from build123d import *

# Parameters (mm, degrees)
SHAPE_DEPTH         = 10.75
CUT_EXTRUDE1_DEPTH  = 6.75
CUT_EXTRUDE2_REACH  = 6
FILLET1_R           = 0.2
SKETCH4_R           = 1
BOSS_EXTRUDE2_DEPTH = 6.1
FILLET2_R           = 1
SKETCH5_W           = 0.2
SKETCH5_H           = 2
SKETCH5_W_2         = 2
SKETCH5_H_2         = 0.2
CUT_EXTRUDE3_DEPTH  = 6.75
CUT_EXTRUDE4_DEPTH  = 2.4
CUT_EXTRUDE5_DEPTH  = 1
SKETCH7_R           = 1.225
SKETCH7_R_2         = 0.625
BOSS_EXTRUDE3_DEPTH = 4
SKETCH9_W           = 1.225
SKETCH9_H           = 2.45
CUT_EXTRUDE6_DEPTH  = 2.3


with BuildPart() as part:
    # Sketch1 → Shape (new body)
    with BuildSketch(Plane(origin=(0, 0, 0), x_dir=(1, 0, 0), z_dir=(0, 1, 0))):
        Polygon((5.075, -1.6), (5.075, 1.6), (4.075, 2.6), (-5.075, 2.6), (-5.075, -2.6), (4.075, -2.6), align=None)
    extrude(amount=SHAPE_DEPTH)

    # Sketch2 → Cut-Extrude1 (cut)
    with BuildSketch(Plane(origin=(0, 10.75, 0), x_dir=(1, 0, 0), z_dir=(0, 1, 0))):
        Polygon((3.826471863, -2), (4.475, -1.351471863), (4.475, 1.351471863), (3.826471863, 2), (-4.475, 2), (-4.475, -2), align=None)
    extrude(amount=-CUT_EXTRUDE1_DEPTH, mode=Mode.SUBTRACT)

    # Sketch3 → Cut-Extrude2 (cut, up to next)
    with BuildSketch(Plane(origin=(0, 4, 0), x_dir=(1, 0, 0), z_dir=(0, 1, 0)), mode=Mode.PRIVATE) as cut_extrude2_sk1:
        with BuildLine():
            Line((-1.675378875, -1.6), (1.675378875, -1.6))
            ThreePointArc((1.675378875, -1.6), (0.7, 0), (1.675378875, 1.6))
            Line((1.675378875, 1.6), (-1.675378875, 1.6))
            ThreePointArc((-1.675378875, 1.6), (-0.963068312, 0.936931688), (-0.7, 0))
            ThreePointArc((-0.7, 0), (-0.963068312, -0.936931688), (-1.675378875, -1.6))
        make_face()
    cut_extrude2_tool1 = extrude(cut_extrude2_sk1.sketch, amount=-CUT_EXTRUDE2_REACH, mode=Mode.PRIVATE) & part.part
    add(cut_extrude2_tool1.solids().sort_by_distance((0, 4, 0))[0], mode=Mode.SUBTRACT)

    # Fillet1
    fillet1_edges = [part.edges().sort_by_distance(p)[0] for p in [
        (1.675378875, 2, 1.6),
        (-1.675378875, 2, 1.6),
        (-1.675378875, 2, -1.6),
        (1.675378875, 2, -1.6),
    ]]
    fillet(fillet1_edges, radius=FILLET1_R)

    # Sketch4 → Boss-Extrude2 (add)
    with BuildSketch(Plane(origin=(0, 4, 0), x_dir=(1, 0, 0), z_dir=(0, 1, 0))):
        with Locations((-2.5, 0)):
            Circle(SKETCH4_R)
        with Locations((2.5, 0)):
            Circle(SKETCH4_R)
    extrude(amount=BOSS_EXTRUDE2_DEPTH)

    # Fillet2
    fillet2_edges = [part.edges().sort_by_distance(p)[0] for p in [
        (-3.5, 10.1, 0),
        (1.5, 10.1, 0),
    ]]
    fillet(fillet2_edges, radius=FILLET2_R)

    # Sketch5 → Cut-Extrude3 (cut)
    with BuildSketch(Plane(origin=(0, 10.75, 0), x_dir=(1, 0, 0), z_dir=(0, 1, 0))):
        with Locations((-2.5, 0)):
            Rectangle(SKETCH5_W, SKETCH5_H)
        with Locations((-2.5, 0)):
            Rectangle(SKETCH5_W_2, SKETCH5_H_2)
        with Locations((2.5, 0)):
            Rectangle(SKETCH5_W_2, SKETCH5_H_2)
        with Locations((2.5, 0)):
            Rectangle(SKETCH5_W, SKETCH5_H)
    extrude(amount=-CUT_EXTRUDE3_DEPTH, mode=Mode.SUBTRACT)

    # Sketch6 → Cut-Extrude4 (cut)
    with BuildSketch(Plane(origin=(0, 0.5, 0), x_dir=(-1, 0, 0), z_dir=(0, -1, 0))):
        Polygon((-5.075, -1.6), (-4.075, -2.6), (5.075, -2.6), (5.075, 2.6), (-4.075, 2.6), (-5.075, 1.6), align=None)
        Polygon((-4.875, -1.517157288), (-3.992157288, -2.4), (4.875, -2.4), (4.875, 2.4), (-3.992157288, 2.4), (-4.875, 1.517157288), align=None, mode=Mode.SUBTRACT)
    extrude(amount=-CUT_EXTRUDE4_DEPTH, mode=Mode.SUBTRACT)

    # Sketch8 → Cut-Extrude5 (cut)
    with BuildSketch(Plane.XZ):
        Polygon((-4.475, -2), (-4.475, 2), (3.826471863, 2), (4.475, 1.351471863), (4.475, -1.351471863), (3.826471863, -2), align=None)
    extrude(amount=-CUT_EXTRUDE5_DEPTH, mode=Mode.SUBTRACT)

    # Sketch7 → Boss-Extrude3 (add)
    with BuildSketch(Plane.XZ.offset(-1)):
        with Locations((-2.5, 0)):
            Circle(SKETCH7_R)
        with Locations((-2.5, 0)):
            Circle(SKETCH7_R_2, mode=Mode.SUBTRACT)
        with Locations((2.5, 0)):
            Circle(SKETCH7_R)
        with Locations((2.5, 0)):
            Circle(SKETCH7_R_2, mode=Mode.SUBTRACT)
    extrude(amount=BOSS_EXTRUDE3_DEPTH)

    # Sketch9 → Cut-Extrude6 (cut)
    with BuildSketch(Plane.XZ.offset(3)):
        with Locations((-3.1125, 0)):
            Rectangle(SKETCH9_W, SKETCH9_H)
        with Locations((3.1125, 0)):
            Rectangle(SKETCH9_W, SKETCH9_H)
    extrude(amount=-CUT_EXTRUDE6_DEPTH, mode=Mode.SUBTRACT)


solid = part.part
The model under review builds one solid part; all positions refer to its coordinate system, in mm. A direction names the side the tool comes from. Round coordinates to 2 decimals unless told otherwise and drop trailing zeros. Loops run counter-clockwise (first coordinate to the right, second up) from the corner with the lowest first, then second, coordinate; pieces in that order, holes last. Notation, with made-up numbers: (20, 58.5) -> (41, 58.5) arc R19 ccw to (41, 64.5) -> close; hole circle Ø4 at (5.5, -28.75). An arc over 180 degrees is marked (long way). One line per question, with ' | ' between items. Start each with the question number.
Item 1: Draft analysis for pull direction Y (two halves, no side actions). For faces 5 (the face through (2.6, 7.1, 0.6)), 6 (the face through (4.44, 1.68, 1.95)), 7 (the face through (3.4, -0.7, 0)), state which applies: +Y half, -Y half, draft (parallel to the pull), parting line (faces both ways), or undercut.
Item 2: Add section A-A, the plane y = 10.25. Write out the cut boundary in (x, z) (3 decimals).
Item 3: Add section B-B, the plane y = 6. Count the separate pieces of the cut face and the enclosed holes in it, then the cut area to 3 significant figures.
Item 4: Add section C-C, the plane z = -2.15. Write out the cut boundary in (x, y) (3 decimals), then the cut area to 3 significant figures.
Item 5: Add section D-D, the plane y = 1.25. Write out the cut boundary in (x, z) (3 decimals), then the cut area to 3 significant figures.
Item 6: Wall thickness on line 1 along X through (y, z) = (-0.45, 0) (3 decimals); line 2 along Z through (x, y) = (-2.5, 0.25) (3 decimals); line 3 along Z through (x, y) = (-4.25, 7.5): over which ranges is each line inside the solid? List them lowest first. Write a range as [from, to].
Item 7: Machinability: for faces 1 (the face through (-2, 7, 0.1)), 2 (the face through (-0.4, 0.5, 2)), 3 (the face through (0.7, 2.5, 0)), 4 (the face through (4.568, 6.77, 2.107)), which of the approach directions +Z, -Z, +X, -X, +Y, -Y give a long, thin tool a straight path to every point of the face, cutting with its end or side? Answer none if there is none.
Item 8: For pin 1 (0.6 mm diameter, centred on x = 3.5, z = 0.5, fed in from -Y); pin 2 (1 mm diameter, centred on y = 1.5, z = -1, fed in from +X) (3 decimals); pin 3 (0.5 mm diameter, centred on y = -1.5, z = -1, fed in from +X), all flat-tipped, find the tip position at first contact; note any pin that passes through.
Return value:
1) face 5: draft | face 6: undercut | face 7: -Y half
2) outline: (-5.075, -2.6) -> (4.075, -2.6) -> (5.075, -1.6) -> (5.075, 1.6) -> (4.075, 2.6) -> (-5.075, 2.6) -> close; hole (-4.475, -2) -> (3.826, -2) -> (4.475, -1.351) -> (4.475, 1.351) -> (3.826, 2) -> (-4.475, 2) -> close
3) separate pieces: 9 | enclosed holes: 1 | area: 21.2 mm2
4) outline: (-5.075, 0) -> (4.525, 0) -> (4.525, 0.5) -> (4.242, 0.5) -> (4.242, 2.9) -> (4.525, 2.9) -> (4.525, 10.75) -> (-5.075, 10.75) -> (-5.075, 2.9) -> (-4.875, 2.9) -> (-4.875, 0.5) -> (-5.075, 0.5) -> close | area: 102 mm2
5) outline: (-4.875, -2.4) -> (3.992, -2.4) -> (4.875, -1.517) -> (4.875, 1.517) -> (3.992, 2.4) -> (-4.875, 2.4) -> close; hole (-1.215, -1.26) arc R0.2 ccw to (-1.072, -1.6) -> (1.072, -1.6) arc R0.2 ccw to (1.215, -1.26) arc R1.8 cw to (1.215, 1.26) arc R0.2 ccw to (1.072, 1.6) -> (-1.072, 1.6) arc R0.2 ccw to (-1.215, 1.26) arc R1.8 cw to start | area: 40.0 mm2
6) line 1: x = [-3.725, -3.125], [-1.875, -1.275], [1.275, 1.875], [3.125, 3.725] | line 2: z = [-2.6, -2], [-1.225, -0.625], [0.625, 1.225], [2, 2.6] | line 3: z = [-2.6, -2], [2, 2.6]
7) face 1: +Y | face 2: -Y | face 3: +Y, -Y | face 4: +Z, +X, +Y, -Y
8) pin 1: stops at y = -0.7 | pin 2: stops at x = 4.875 | pin 3: stops at x = 2.5
